from build123d import *

# Parameters (mm, degrees)
SKETCH_1_R            = 6.5
EXTRUDE_255_DEPTH     = 8
CUT_EXTRUDE_389_DEPTH = 4
SKETCH_3_R            = 4
EXTRUDE_494_DEPTH     = 65
SKETCH_4_R            = 3
EXTRUDE_M6_DEPTH      = 10


with BuildPart() as part:
    # 草图1 → Extrude 255 (new body)
    with BuildSketch(Plane(origin=(0, 0, 0), x_dir=(1, 0, 0), z_dir=(0, 1, 0))):
        Circle(SKETCH_1_R)
    extrude(amount=EXTRUDE_255_DEPTH)

    # 草图2 → Cut-Extrude 389 (cut)
    with BuildSketch(Plane(origin=(0, 8, 0), x_dir=(1, 0, 0), z_dir=(0, 1, 0))):
        Polygon((3.579571669, 0), (1.789785834, 3.1), (-1.789785834, 3.1), (-3.579571669, 0), (-1.789785834, -3.1), (1.789785834, -3.1), align=None)
    extrude(amount=-CUT_EXTRUDE_389_DEPTH, mode=Mode.SUBTRACT)

    # 草图3 → Extrude 494 (add)
    with BuildSketch(Plane.XZ):
        Circle(SKETCH_3_R)
    extrude(amount=EXTRUDE_494_DEPTH)

    # 草图4 → M6螺纹 (add)
    with BuildSketch(Plane.XZ.offset(65)):
        Circle(SKETCH_4_R)
    extrude(amount=EXTRUDE_M6_DEPTH)


solid = part.part
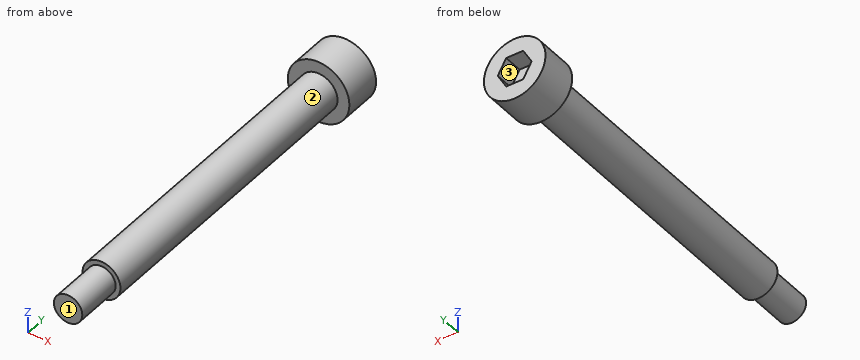
Source: CAD feature listing. Evaluate the final solid. Frame: model axes, mm. Face numbers are marked on the shaded views. A direction names the side the tool comes from. Round coordinates to 2 decimals unless told otherwise and drop trailing zeros. Loops run counter-clockwise (first coordinate to the right, second up) from the corner with the lowest first, then second, coordinate; pieces in that order, holes last. Notation, with made-up numbers: M 28,77 L 86,77 A23 cw 86,116 Z; hole C 17.25,-13 d11. An arc over 180 degrees is marked long. Return JSON: item names as keys, results as strings. Group by question number.
1. Reachability of the marked faces 1, 2 and 3 from +Z, -Z, +X, -X, +Y, -Y: full face, straight path, thin tool, end or side. Return the list, or none.
2. Material intervals for line 1 along X through (y, z) = (-10.5, 1.75); line 2 along Y through (x, z) = (0.5, -0.25); line 3 along Z through (x, y) = (0, -33), sorted ascending. Write a range as from..to.
3. Section query A-A on x = 0. Output: boundary loops of the cut face in (y, z), and give its area (3 significant figures).
4. Section query B-B on y = -7. Output: boundary loops of the cut face in (x, z).
5. Pin query (flat end, axial travel): pin 1 (1.5 mm diameter, centred on x = 4, y = -22.5, fed in from -Z); pin 2 (5 mm diameter, centred on y = -23.5, z = 2, fed in from -X); pin 3 (6 mm diameter, centred on x = 3, y = -7.5, fed in from +Z). Return the tip coordinate at first contact, or that it passes through.
6. Section query C-C on z = 2. Output: boundary loops of the cut face in (x, y).
Checks:
{
 "1": {"face 1": "+Z, -Z, +X, -X, -Y", "face 2": "-Y", "face 3": "+Y"},
 "2": {"line 1": "x = -3.6..3.6", "line 2": "y = -75..4", "line 3": "z = -4..4"},
 "3": {"outline": "M -75,-3 L -65,-3 L -65,-4 L 0,-4 L 0,-6.5 L 8,-6.5 L 8,-3.1 L 4,-3.1 L 4,3.1 L 8,3.1 L 8,6.5 L 0,6.5 L 0,4 L -65,4 L -65,3 L -75,3 Z", "area": "659 mm²"},
 "4": {"outline": "C 0,0 d8"},
 "5": {"pin 1": "stops at z = -2.33", "pin 2": "stops at x = -4", "pin 3": "stops at z = 4"},
 "6": {"outline": "M -6.18,0 L -3.46,0 L -3.46,-65 L -2.24,-65 L -2.24,-75 L 2.24,-75 L 2.24,-65 L 3.46,-65 L 3.46,0 L 6.18,0 L 6.18,8 L 2.42,8 L 2.42,4 L -2.42,4 L -2.42,8 L -6.18,8 Z"}
}
